from build123d import *

# Parameters (mm, degrees)
BOSS_EXTRUDE1_DEPTH     = 120
SKETCH5_R               = 5
BOSS_EXTRUDE2_DEPTH     = 20
FILLET1_R               = 1.5
SKETCH7_R               = 5
CUT_EXTRUDE1_DEPTH      = 57
CUT_EXTRUDE1_DEPTH_BACK = 47


with BuildPart() as part:
    # Sketch2 → Boss-Extrude1 (new body)
    with BuildSketch(Plane.XY):
        Polygon((0, 0), (10, 0), (10, 40), (13, 40), (16, -20), (-6, -20), (-3, 40), (0, 40), align=None)
    extrude(amount=-BOSS_EXTRUDE1_DEPTH)

    # Sketch5 → Boss-Extrude2 (add)
    with BuildSketch(Plane.XZ.offset(20)):
        with BuildLine():
            Line((16, -50), (46, -50))
            ThreePointArc((46, -50), (56, -60), (46, -70))
            Line((46, -70), (16, -70))
            Line((16, -70), (13, -70))
            Line((13, -70), (13, -50))
            Line((13, -50), (16, -50))
        make_face()
        with Locations((46, -60)):
            Circle(SKETCH5_R, mode=Mode.SUBTRACT)
        with BuildLine():
            Line((-6, -50), (-36, -50))
            ThreePointArc((-36, -50), (-46, -60), (-36, -70))
            Line((-36, -70), (-6, -70))
            Line((-6, -70), (-3, -70))
            Line((-3, -70), (-3, -50))
            Line((-3, -50), (-6, -50))
        make_face()
        with Locations((-36, -60)):
            Circle(SKETCH5_R, mode=Mode.SUBTRACT)
    extrude(amount=-BOSS_EXTRUDE2_DEPTH)

    # Fillet1
    fillet1_edges = [part.edges().sort_by_distance(p)[0] for p in [
        (15.5, -10, -50),
        (15.5, -10, -70),
        (-5.5, -10, -50),
        (-5.5, -10, -70),
    ]]
    fillet(fillet1_edges, radius=FILLET1_R)

    # Sketch7 → Cut-Extrude1 (cut, two sides)
    with BuildSketch(Plane(origin=(0, 0, 0), x_dir=(0, 0, -1), z_dir=(1, 0, 0))) as cut_extrude1_sk:
        with Locations((15, 25)):
            Circle(SKETCH7_R)
        with Locations((105, 25)):
            Circle(SKETCH7_R)
    extrude(amount=CUT_EXTRUDE1_DEPTH, mode=Mode.SUBTRACT)
    extrude(cut_extrude1_sk.sketch, amount=-CUT_EXTRUDE1_DEPTH_BACK, mode=Mode.SUBTRACT)


solid = part.part
Could you check a few things on this model? Use its own coordinates, in mm. A direction names the side the tool comes from. Give positions to 0.01 mm unless a question says otherwise; leave off trailing zeros. Order: outer loops, then holes, each group sorted by start corner. A loop starts at its lowest first (then second) coordinate and runs counter-clockwise, first axis right, second up.
1. Suppose I cut it at C-C (y = 17). List the corners of the cut face in (x, z) for me.
2. Suppose I cut it at D-D (z = -89.5). List the corners of the cut face in (x, y) for me, plus the area to 3 significant figures.
3. For faces 4 (the flat face through (5, -3, 0)), 5 (the flat face through (14.48, 10.42, -59.16)), 6 (the flat face through (0, 20, -59)), which set-ups out of +Z, -Z, +X, -X, +Y, -Y let a thin tool reach every point of the face, with its end or its side?
4. I need wall thicknesses on L1, parallel to Z at x = 12.7, y = 25; L2, parallel to Z at x = -36, y = -4.25; L3, parallel to X at y = -17, z = -57. Which ranges of each line are inside material? Lowest first, please.
5. Suppose I cut it at B-B (z = -105). List the corners of the cut face in (x, y) for me.
6. Suppose I cut it at A-A (y = 25). List the corners of the cut face in (x, z) for me.
7. We'd pull the mould along Z, two halves only. Please class faces 1 (the cylindrical face through (11.997, 20.564, -107.307)), 2 (the cylindrical face through (-46, -10, -60)), 3 (the flat face through (36, 0, -60)): pulls with the +Z half, pulls with the -Z half, needs draft (parallel to the pull), parting line crosses it, or undercut.
8. Will these pins go through, and if not, where does the flat tip stop? P1, Ø16, axis at x = 28, y = -13.5, coming from the -Z side; P2, Ø11.5, axis at x = 42.5, z = -61.5, coming from the +Y side; P3, Ø4, axis at y = 2.5, z = -32.5, coming from the -X side (3 decimals).
Solved:
1. outline: (-4.15, -120) - (0, -120) - (0, 0) - (-4.15, 0) - close; (10, -120) - (14.15, -120) - (14.15, 0) - (10, 0) - close
2. outline: (-6, -20) - (16, -20) - (13, 40) - (10, 40) - (10, 0) - (0, 0) - (0, 40) - (-3, 40) - close
2. area: 740 mm2
3. face 4: +Z, +X, -X, +Y, -Y
3. face 5: +X, +Y
3. face 6: +Z, -Z, +Y
4. L1: z = -120 to -110, -100 to -20, -10 to 0
4. L2: z = -70 to -65, -55 to -50
4. L3: x = -45.54 to -40, -32 to 42, 50 to 55.54
5. outline: (-6, -20) - (16, -20) - (14, 20) - (10, 20) - (10, 0) - (0, 0) - (0, 20) - (-4, 20) - close; (-3.5, 30) - (0, 30) - (0, 40) - (-3, 40) - close; (10, 30) - (13.5, 30) - (13, 40) - (10, 40) - close
6. outline: (-3.75, -120) - (0, -120) - (0, -110) - (-3.75, -110) - close; (-3.75, -100) - (0, -100) - (0, -20) - (-3.75, -20) - close; (-3.75, -10) - (0, -10) - (0, 0) - (-3.75, 0) - close; (10, -120) - (13.75, -120) - (13.75, -110) - (10, -110) - close; (10, -100) - (13.75, -100) - (13.75, -20) - (10, -20) - close; (10, -10) - (13.75, -10) - (13.75, 0) - (10, 0) - close
7. face 1: undercut
7. face 2: parting line crosses it
7. face 3: needs draft
8. P1: stops at z = -70
8. P2: stops at y = 0
8. P3: stops at x = -4.975
